from build123d import *

# Parameters (mm, degrees)
F0_W     = 81.7696005106
F0_H     = 43.3689393103
F1_DEPTH = 25.4
F3_D     = 6.35
F3_DEPTH = 12.7
F3_TIP   = 1.9077324654
F5_SIZE  = 5.08


# Not quite as in the source:
# - the program builds the solid bodies; features that only make, move or delete a surface that nothing else refers to are left out


with BuildPart() as f1:
    # F0 (on Front) → F1 (new body)
    with BuildSketch(Plane.XZ):
        with Locations((-0.1035071909, 21.6844696552)):
            Rectangle(F0_W, F0_H)
    extrude(amount=-F1_DEPTH)

    # F3
    with Locations(Plane.XZ):
        with Locations((36.8480719626, 4.8647737131), (-36.8480719626, 5.071785301)):
            Hole(F3_D / 2, depth=F3_DEPTH)
            with Locations((0, 0, -(F3_DEPTH + F3_TIP / 2))):  # 118° drill point
                Cone(0, F3_D / 2, F3_TIP, mode=Mode.SUBTRACT)

    # F5
    f5_edges = [f1.edges().sort_by_distance(p)[0] for p in [
        (-40.988307, 25.4, 21.68447),
        (-0.103507, 25.4, 0),
        (40.781293, 25.4, 21.68447),
        (-0.103507, 25.4, 43.368939),
    ]]
    chamfer(f5_edges, length=F5_SIZE)


solid = f1.part
Geometry: final body of the model. Coordinates: model frame, mm. A direction names the side the tool comes from. Coordinates: 2 decimals unless noted, no trailing zeros. Loops run counter-clockwise (first coordinate to the right, second up) from the corner with the lowest first, then second, coordinate; pieces in that order, holes last. Notation, with made-up numbers: (21, 64.5) - (62, 64.5) arc R15 cw to (62, 83.5) - close; hole circle Ø6 at (57.5, 20.5). An arc over 180 degrees is marked (long way). One line per question, with ' | ' between items. Start each with the question number.
(1) Draft query along X for faces 3 (the flat face through (-0.68, 22.9, 2.58)), 4 (the flat face through (-38.41, 22.9, 21.38)), 5 (the flat face through (40.781, 10, 21)), 6 (the conical face through (37.357, 14.276, 4.654)). Return one class per face: +X half, -X half, draft (parallel to the pull), parting line (faces both ways), or undercut.
(2) Ray query, L1, parallel to Z at x = 37, y = 3.75; L2, parallel to X at y = 9.5, z = 2.5; L3, parallel to X at y = 4.75, z = 5.5. Return the intervals inside material, ascending. Write a range as from..to.
(3) Cut plane B-B on y = 10.5. Output: boundary loops of the cut face in (x, z) (3 decimals).
(4) First-contact query: pin 1 (12 mm diameter, centred on x = 26.5, z = 21, fed in from -Y); pin 2 (5 mm diameter, centred on x = 36.85, z = 4.86, fed in from -Y). Flat tips, straight axial feed; report the tip coordinate or a pass-through.
(5) Reachability of faces 1 (the flat face through (-1, 10, 43.369)), 2 (the cylindrical face through (33.82, 6.44, 5.82)) from +Z, -Z, +X, -X, +Y, -Y: full face, straight path, thin tool, end or side. Return the list, or none.
(6) Cut plane A-A on x = -29.5. Output: boundary loops of the cut face in (y, z).
Here are the results:
1) face 3: draft | face 4: -X half | face 5: +X half | face 6: undercut
2) L1: 0..1.69, 8.04..43.37 | L2: -40.99..-38.71, -34.99..34.73, 38.97..40.78 | L3: -40.99..-39.99, -33.7..33.74, 39.96..40.78
3) outline: (-40.988, 0) - (40.781, 0) - (40.781, 43.369) - (-40.988, 43.369) - close; hole circle Ø6.35 at (-36.848, 5.072); hole circle Ø6.35 at (36.848, 4.865)
4) pin 1: y = 0 | pin 2: y = 13.1
5) face 1: +Z, +X, -X, +Y, -Y | face 2: -Y
6) outline: (0, 0) - (20.32, 0) - (25.4, 5.08) - (25.4, 38.29) - (20.32, 43.37) - (0, 43.37) - close
